Part model, mm, in its own coordinate system. Face numbers are marked on the shaded views. A direction names the side the tool comes from. Give positions to 0.01 mm unless a question says otherwise; leave off trailing zeros. Write each loop counter-clockwise with the first axis right and the second up, starting at its lowest first coordinate (ties: lowest second). Pieces come first, ordered by that corner, then holes. Notation, with made-up numbers: (57, 5) - (92, 5) arc R15 cw to (92, 13) - close; hole circle Ø4 at (-31.75, 45.25). An arc over 180 degrees is marked (long way). Answer as a JSON object with one key per item and string values. Group by question number.
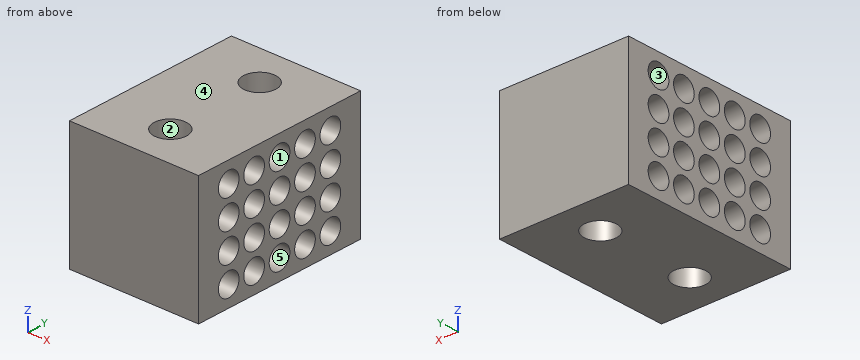
```python
from build123d import *

# Parameters (mm, degrees)
F0_W     = 20.32
F0_H     = 28.32
F0_R     = 2.54
F1_DEPTH = 19.685
F2_R     = 1.80975
F3_DEPTH = 5.08
F4_R     = 1.80975
F5_DEPTH = 5.08


with BuildPart() as f1:
    # F0 (on Top) → F1 (new body)
    with BuildSketch(Plane.XY):
        with Locations((-10.16, 14.16)):
            Rectangle(F0_W, F0_H)
        with Locations((-10.16, 6.349)):
            Circle(F0_R, mode=Mode.SUBTRACT)
        with Locations((-10.16, 21.97)):
            Circle(F0_R, mode=Mode.SUBTRACT)
    extrude(amount=F1_DEPTH)

    # F2 (on face) → F3 (cut)
    with BuildSketch(Plane.YZ):
        with Locations((5.2705, 16.51)):
            Circle(F2_R)
        with Locations((9.7155, 16.51)):
            Circle(F2_R)
        with Locations((14.1605, 16.51)):
            Circle(F2_R)
        with Locations((18.6055, 16.51)):
            Circle(F2_R)
        with Locations((23.0505, 16.51)):
            Circle(F2_R)
        with Locations((23.0505, 12.065)):
            Circle(F2_R)
        with Locations((18.6055, 12.065)):
            Circle(F2_R)
        with Locations((14.1605, 12.065)):
            Circle(F2_R)
        with Locations((9.7155, 12.065)):
            Circle(F2_R)
        with Locations((5.2705, 12.065)):
            Circle(F2_R)
        with Locations((23.0505, 7.62)):
            Circle(F2_R)
        with Locations((18.6055, 7.62)):
            Circle(F2_R)
        with Locations((14.1605, 7.62)):
            Circle(F2_R)
        with Locations((9.7155, 7.62)):
            Circle(F2_R)
        with Locations((5.2705, 7.62)):
            Circle(F2_R)
        with Locations((23.0505, 3.175)):
            Circle(F2_R)
        with Locations((18.6055, 3.175)):
            Circle(F2_R)
        with Locations((14.1605, 3.175)):
            Circle(F2_R)
        with Locations((9.7155, 3.175)):
            Circle(F2_R)
        with Locations((5.2705, 3.175)):
            Circle(F2_R)
    extrude(amount=-F3_DEPTH, mode=Mode.SUBTRACT)

    # F4 (on face) → F5 (cut)
    with BuildSketch(Plane(origin=(-20.32, 0, 0), x_dir=(0, -1, 0), z_dir=(-1, 0, 0))):
        with Locations((-23.084547, 16.517471)):
            Circle(F4_R)
        with Locations((-18.639547, 16.517471)):
            Circle(F4_R)
        with Locations((-14.194547, 16.517471)):
            Circle(F4_R)
        with Locations((-9.749547, 16.517471)):
            Circle(F4_R)
        with Locations((-5.304547, 16.517471)):
            Circle(F4_R)
        with Locations((-5.304547, 12.072471)):
            Circle(F4_R)
        with Locations((-9.749547, 12.072471)):
            Circle(F4_R)
        with Locations((-14.194547, 12.072471)):
            Circle(F4_R)
        with Locations((-18.639547, 12.072471)):
            Circle(F4_R)
        with Locations((-23.084547, 12.072471)):
            Circle(F4_R)
        with Locations((-5.304547, 7.627471)):
            Circle(F4_R)
        with Locations((-9.749547, 7.627471)):
            Circle(F4_R)
        with Locations((-14.194547, 7.627471)):
            Circle(F4_R)
        with Locations((-18.639547, 7.627471)):
            Circle(F4_R)
        with Locations((-23.084547, 7.627471)):
            Circle(F4_R)
        with Locations((-5.304547, 3.182471)):
            Circle(F4_R)
        with Locations((-9.749547, 3.182471)):
            Circle(F4_R)
        with Locations((-14.194547, 3.182471)):
            Circle(F4_R)
        with Locations((-18.639547, 3.182471)):
            Circle(F4_R)
        with Locations((-23.084547, 3.182471)):
            Circle(F4_R)
    extrude(amount=-F5_DEPTH, mode=Mode.SUBTRACT)


solid = f1.part
```
1) Probe line 1 (Y direction, x = -17.5, z = 16.5); line 2 (Z direction, x = -18.25, y = 18.5) (3 decimals); line 3 (X direction, y = 6.5, z = 3). List the from-to ranges inside material, lowest first.
2) Drop flat-ended pins along their axis: P1, Ø4, axis at y = 9.75, z = 16.52, coming from the +X side; P2, Ø1.8, axis at y = 14, z = 17, coming from the -X side; P3, Ø3.5, axis at y = 18.61, z = 16.51, coming from the +X side. Give the stop position or say it passes through.
3) Band-saw the part on B-B (x = -18). State how many separate pieces and enclosed holes the cut face has, plus the area to 3 significant figures.
4) Band-saw the part on A-A (x = -10.16). List the corners of the cut face in (y, z) (3 decimals), plus the area to 3 significant figures.
5) Which spindle directions (+Z, -Z, +X, -X, +Y, -Y) get a long thin tool onto all of the face, cutting with end or side? Do the marked faces 3, 4 and 5. Say none if no direction does.
6) Mould opens along X. For the marked faces 1 and 2 say: pulls with the +X half, pulls with the -X half, needs draft (parallel to the pull), parting line crosses it, or undercut.
Verdict:
{
 "1": {"line 1": "0 to 3.49, 7.11 to 7.94, 11.56 to 12.38, 16 to 16.83, 20.45 to 21.27, 24.89 to 28.32", "line 2": "0 to 1.378, 4.987 to 5.823, 9.432 to 10.268, 13.877 to 14.713, 18.322 to 19.685", "line 3": "-15.24 to -12.7, -7.62 to -5.08"},
 "2": {"P1": "x = 0", "P2": "x = -15.24", "P3": "x = -5.08"},
 "3": {"separate pieces": "1", "enclosed holes": "20", "area": "352 mm2"},
 "4": {"outline": "(0, 0) - (3.809, 0) - (3.809, 19.685) - (0, 19.685) - close; (8.889, 0) - (19.43, 0) - (19.43, 19.685) - (8.889, 19.685) - close; (24.51, 0) - (28.32, 0) - (28.32, 19.685) - (24.51, 19.685) - close", "area": "357 mm2"},
 "5": {"face 3": "-X", "face 4": "+Z, +X, -X, +Y, -Y", "face 5": "+X"},
 "6": {"face 1": "needs draft", "face 2": "undercut"}
}
